```python
from build123d import *
from OCP.BRepFilletAPI import BRepFilletAPI_MakeChamfer

# Parameters (mm, degrees)
BOSS_EXTRUDE3_DEPTH            = 10
SKETCH13_W                     = 10
SKETCH13_H                     = 12
BOSS_EXTRUDE5_DEPTH            = 20
SKETCH15_R                     = 2.55
CUT_EXTRUDE7_DEPTH             = 82.299792521
CBORE_FOR_M4_SHCS1_D           = 4.5
CBORE_FOR_M4_SHCS1_DEPTH       = 15.5
CBORE_FOR_M4_SHCS1_CBORE_D     = 8
CBORE_FOR_M4_SHCS1_CBORE_DEPTH = 4
CBORE_FOR_M4_SHCS1_TIP         = 1.351936393
SKETCH21_R                     = 1.118017303
BOSS_EXTRUDE6_DEPTH            = 1
CIRPATTERN3_COUNT              = 3
SKETCH22_R                     = 1.118017303
CUT_EXTRUDE8_DEPTH             = 1
FILLET1_R                      = 4
CHAMFER1_SIZE                  = 1
CHAMFER1_SIZE2                 = 1.227870321
CHAMFER2_SIZE                  = 1
CHAMFER2_SIZE2                 = 0.307449129


with BuildPart() as part:
    # Sketch6 → Boss-Extrude3 (new body)
    with BuildSketch(Plane(origin=(0, 0, 0), x_dir=(1, 0, 0), z_dir=(0, 1, 0))):
        with BuildLine():
            Line((-40, 33.094010768), (40, 33.094010768))
            ThreePointArc((40, 33.094010768), (48.660254038, 28.094010768), (48.660254038, 18.094010768))
            Line((48.660254038, 18.094010768), (28.660254038, -16.547005384))
            Line((28.660254038, -16.547005384), (8.660254038, -51.188021535))
            ThreePointArc((8.660254038, -51.188021535), (0, -56.188021535), (-8.660254038, -51.188021535))
            Line((-8.660254038, -51.188021535), (-28.660254038, -16.547005384))
            Line((-28.660254038, -16.547005384), (-48.660254038, 18.094010768))
            ThreePointArc((-48.660254038, 18.094010768), (-48.660254038, 28.094010768), (-40, 33.094010768))
        make_face()
    extrude(amount=BOSS_EXTRUDE3_DEPTH)

    # Sketch13 → Boss-Extrude5 (add)
    with BuildSketch(Plane(origin=(0, 0, 0), x_dir=(-1, 0, 0), z_dir=(0, -1, 0))):
        with Locations((-0.25, 20.094010768)):
            Rectangle(SKETCH13_W, SKETCH13_H)
    boss_extrude5 = extrude(amount=BOSS_EXTRUDE5_DEPTH)

    # Sketch15 → Cut-Extrude7 (cut, through all)
    with BuildSketch(Plane(origin=(5.25, 0, 0), x_dir=(0, 0, -1), z_dir=(1, 0, 0))):
        with Locations((20.094010768, -8)):
            Circle(SKETCH15_R)
        with BuildLine():
            Line((14.094010768, -8), (14.094010768, -20))
            Line((14.094010768, -20), (26.094010768, -20))
            Line((26.094010768, -20), (26.094010768, -8))
            ThreePointArc((26.094010768, -8), (20.094010768, -14), (14.094010768, -8))
        make_face()
    cut_extrude7 = extrude(amount=-CUT_EXTRUDE7_DEPTH, mode=Mode.SUBTRACT)

    # CBORE for M4 SHCS1
    with Locations(Plane(origin=(0, 0, 0), x_dir=(-1, 0, 0), z_dir=(0, -1, 0))):
        with Locations((-40, 23.094010768), (40, 23.094010768), (0, -46.188021535)):
            CounterBoreHole(CBORE_FOR_M4_SHCS1_D / 2, CBORE_FOR_M4_SHCS1_CBORE_D / 2, CBORE_FOR_M4_SHCS1_CBORE_DEPTH, depth=CBORE_FOR_M4_SHCS1_DEPTH)
            with Locations((0, 0, -(CBORE_FOR_M4_SHCS1_DEPTH + CBORE_FOR_M4_SHCS1_TIP / 2))):  # 118° drill point
                Cone(0, CBORE_FOR_M4_SHCS1_D / 2, CBORE_FOR_M4_SHCS1_TIP, mode=Mode.SUBTRACT)

    # Sketch21 → Boss-Extrude6 (add)
    with BuildSketch(Plane(origin=(0, 0, 0), x_dir=(-1, 0, 0), z_dir=(0, -1, 0))):
        with Locations(Location((0, 0, 0), (0, 0, 270))):
            Circle(SKETCH21_R)
    boss_extrude6 = extrude(amount=BOSS_EXTRUDE6_DEPTH)

    # CirPattern3: Boss-Extrude5, Cut-Extrude7, Boss-Extrude6 ×3 about axis
    cirpattern3_axis = Axis((0, 0, 0), (0, 1, 0))
    add([boss_extrude5.rotate(cirpattern3_axis, i * 360 / CIRPATTERN3_COUNT) for i in range(1, CIRPATTERN3_COUNT)])
    add([cut_extrude7.rotate(cirpattern3_axis, i * 360 / CIRPATTERN3_COUNT) for i in range(1, CIRPATTERN3_COUNT)], mode=Mode.SUBTRACT)
    add([boss_extrude6.rotate(cirpattern3_axis, i * 360 / CIRPATTERN3_COUNT) for i in range(1, CIRPATTERN3_COUNT)])

    # Sketch22 → Cut-Extrude8 (cut)
    with BuildSketch(Plane(origin=(0, -1, 0), x_dir=(-1, 0, 0), z_dir=(0, -1, 0))):
        Circle(SKETCH22_R)
    extrude(amount=-CUT_EXTRUDE8_DEPTH, mode=Mode.SUBTRACT)

    # Fillet1
    fillet1_edges = [part.edges().sort_by_distance(p)[0] for p in [
        (-12.330771366, 0, 6.830499033),
        (-15.026923789, 0, 14.160626052),
        (-22.723076211, 0, 12.830499033),
        (-20.026923789, 0, 5.500372014),
        (0.25, 0, -14.094010768),
        (-4.75, 0, -20.094010768),
        (0.25, 0, -26.094010768),
        (5.25, 0, -20.094010768),
        (12.080771366, 0, 7.263511735),
        (19.776923789, 0, 5.933384716),
        (22.473076211, 0, 13.263511735),
        (14.776923789, 0, 14.593638754),
    ]]
    fillet(fillet1_edges, radius=FILLET1_R)

    # Chamfer1: one chamfer whose edges measure the first distance from different faces: ONE call of the kernel's chamfer builder (chamfer() names one face for all edges)
    chamfer1_edges_1 = [part.edges().sort_by_distance(p)[0] for p in [
        (-48.660254038, 10, -28.094010768),
    ]]
    chamfer1_side_1 = [part.faces().sort_by_distance(p)[0] for p in [
        (-48.660254038, 5, -28.094010768),
    ]]
    chamfer1_edges_2 = [part.edges().sort_by_distance(p)[0] for p in [
        (-28.660254038, 10, 16.547005384),
    ]]
    chamfer1_side_2 = [part.faces().sort_by_distance(p)[0] for p in [
        (-28.660254038, 5, 16.547005384),
    ]]
    chamfer1_edges_3 = [part.edges().sort_by_distance(p)[0] for p in [
        (0, 10, 56.188021535),
    ]]
    chamfer1_side_3 = [part.faces().sort_by_distance(p)[0] for p in [
        (0, 5, 56.188021535),
    ]]
    chamfer1_edges_4 = [part.edges().sort_by_distance(p)[0] for p in [
        (28.660254038, 10, 16.547005384),
    ]]
    chamfer1_side_4 = [part.faces().sort_by_distance(p)[0] for p in [
        (28.660254038, 5, 16.547005384),
    ]]
    chamfer1_edges_5 = [part.edges().sort_by_distance(p)[0] for p in [
        (48.660254038, 10, -28.094010768),
    ]]
    chamfer1_side_5 = [part.faces().sort_by_distance(p)[0] for p in [
        (48.660254038, 5, -28.094010768),
    ]]
    chamfer1_edges_6 = [part.edges().sort_by_distance(p)[0] for p in [
        (0, 10, -33.094010768),
    ]]
    chamfer1_side_6 = [part.faces().sort_by_distance(p)[0] for p in [
        (0, 5, -33.094010768),
    ]]
    chamfer1 = BRepFilletAPI_MakeChamfer(part.part.solid().wrapped)
    for e in chamfer1_edges_1:
        chamfer1.Add(CHAMFER1_SIZE, CHAMFER1_SIZE2, e.wrapped, chamfer1_side_1[0].wrapped)  # the first distance lies on this face
    for e in chamfer1_edges_2:
        chamfer1.Add(CHAMFER1_SIZE, CHAMFER1_SIZE2, e.wrapped, chamfer1_side_2[0].wrapped)  # the first distance lies on this face
    for e in chamfer1_edges_3:
        chamfer1.Add(CHAMFER1_SIZE, CHAMFER1_SIZE2, e.wrapped, chamfer1_side_3[0].wrapped)  # the first distance lies on this face
    for e in chamfer1_edges_4:
        chamfer1.Add(CHAMFER1_SIZE, CHAMFER1_SIZE2, e.wrapped, chamfer1_side_4[0].wrapped)  # the first distance lies on this face
    for e in chamfer1_edges_5:
        chamfer1.Add(CHAMFER1_SIZE, CHAMFER1_SIZE2, e.wrapped, chamfer1_side_5[0].wrapped)  # the first distance lies on this face
    for e in chamfer1_edges_6:
        chamfer1.Add(CHAMFER1_SIZE, CHAMFER1_SIZE2, e.wrapped, chamfer1_side_6[0].wrapped)  # the first distance lies on this face
    add(Compound.cast(chamfer1.Shape()), mode=Mode.REPLACE)

    # Chamfer2
    chamfer2_edges = [part.edges().sort_by_distance(p)[0] for p in [
        (-48.660254038, 0, -28.094010768),
        (0, 0, -33.094010768),
        (48.660254038, 0, -28.094010768),
        (28.660254038, 0, 16.547005384),
        (0, 0, 56.188021535),
        (-28.660254038, 0, 16.547005384),
    ]]
    chamfer2_side = [part.faces().sort_by_distance(p)[0] for p in [
        (0, 0, 0),
    ]]
    chamfer(chamfer2_edges, length=CHAMFER2_SIZE, length2=CHAMFER2_SIZE2, reference=chamfer2_side[0])


solid = part.part
```
CAD build for the part. Positions are in the model's coordinates, mm. A direction names the side the tool comes from. Give positions to 0.01 mm unless a question says otherwise; leave off trailing zeros. Order: outer loops, then holes, each group sorted by start corner. A loop starts at its lowest first (then second) coordinate and runs counter-clockwise, first axis right, second up.
(1) Tool access for faces 1 (the cylindrical face through (10.64, -0.7, 6.28)), 2 (the cylindrical face through (-14.28, -0.7, 15.74)), 3 (the flat face through (19.7, -11.15, 5.89)), 4 (the flat face through (-4.75, -11, -20)): list every direction of +Z, -Z, +X, -X, +Y, -Y with a clear straight run to the whole face (end or side of a thin tool).
(2) Drill centre lines: L1, parallel to Z at x = 0, y = 7.6; L2, parallel to X at y = 2.25, z = -21; L3, parallel to Y at x = -15, z = -9.5. Where is each one in solid material? Low to high.
(3) Mould opens along Z. For faces 5 (the cylindrical face through (14.03, -0.7, 16.17)), 6 (the flat face through (38, 4, -21)), 7 (the cylindrical face through (-17.7, -14, 9.8)) say: released by +Z, released by -Z, zero draft, split by the parting line, or undercut.
(4) Saw through at B-B, the plane y = 2. Give the cut face in (x, z).
(5) Saw through at C-C, the plane x = 34.5. Give the cut face in (y, z).
(6) Flat gauge pins, fed straight in: pin 1 (5 mm diameter, centred on y = -10.5, z = -22.5, fed in from +X); pin 2 (4.5 mm diameter, centred on x = 2, y = -6, fed in from +Z); pin 3 (9 mm diameter, centred on x = 0.5, z = 47.5, fed in from -Y). Where does each tip first touch, or does it go through?
(7) Saw through at A-A, the plane x = 0. Give the cut face in (y, z).
Results found:
1. face 1: -Y
1. face 2: +Z, -Y
1. face 3: -Z, +X, -Y
1. face 4: +Z, -Z, -X, -Y
2. L1: z = -33.09 to 43.94, 48.44 to 56.19
2. L2: x = -49.78 to -43.41, -36.59 to 36.59, 43.41 to 49.78
2. L3: y = 0 to 10
3. face 5: released by +Z
3. face 6: undercut
3. face 7: split by the parting line
4. outline: (-48.66, -18.09) arc R10 ccw to (-40, -33.09) - (40, -33.09) arc R10 ccw to (48.66, -18.09) - (8.66, 51.19) arc R10 ccw to (-8.66, 51.19) - close; hole circle Ø8 at (-40, -23.09); hole circle Ø8 at (0, 46.19); hole circle Ø8 at (40, -23.09)
5. outline: (0, -32.09) - (0.31, -33.09) - (9, -33.09) - (10, -31.87) - (10, 3.98) - (9, 6.43) - (0.31, 6.43) - (0, 4.43) - close
6. pin 1: stops at x = 5.25
6. pin 2: stops at z = -14.09
6. pin 3: stops at y = 0
7. outline: (-8, -26.09) - (-4, -26.09) arc R4 cw to (0, -30.09) - (0, -32.09) - (0.31, -33.09) - (9, -33.09) - (10, -31.87) - (10, 43.94) - (4, 43.94) - (4, 42.19) - (0, 42.19) - (0, -10.09) arc R4 cw to (-4, -14.09) - (-8, -14.09) arc R6 ccw to start; (0, 50.19) - (4, 50.19) - (4, 48.44) - (10, 48.44) - (10, 54.96) - (9, 56.19) - (0.31, 56.19) - (0, 55.19) - close; hole circle Ø5.1 at (-8, -20.09)
